Part model, mm, in its own coordinate system. Face numbers are marked on the shaded views. A direction names the side the tool comes from. Coordinates: 2 decimals unless noted, no trailing zeros. Write each loop counter-clockwise with the first axis right and the second up, starting at its lowest first coordinate (ties: lowest second). Pieces come first, ordered by that corner, then holes. Notation, with made-up numbers: (12, -3) -> (71, -3) arc R19 cw to (71, 32) -> close; hole circle Ø7 at (9.5, 22). An arc over 180 degrees is marked (long way). One line per question, with ' | ' between items. Start each with the question number.
Item 1: Saw through at B-B (x = 0). List the corners of the cut face in (y, z).
Item 2: Probe probe 1 along X at (y, z) = (0.85, 0); probe 2 along Z at (x, y) = (0, 1); probe 3 along X at (y, z) = (0.75, -5.5). List the from-to ranges inside material, lowest first. Write a range as [from, to].
Item 3: Two-plate mould, pull along X, no slides. Class the marked faces 1, 2 and 3: pulls with the +X half, pulls with the -X half, needs draft (parallel to the pull), parting line crosses it, or undercut.
Item 4: Saw through at C-C (y = 1.45). List the corners of the cut face in (x, z), and give its area (3 significant figures).
Item 5: 3-axis set-ups, long thin cutter, end or side, ignore diameter. For the marked faces 4 and 5: which of +Z, -Z, +X, -X, +Y, -Y reach the whole face in a straight line?
Item 6: Saw through at A-A (z = 0). List the corners of the cut face in (x, y).
Item 7: Pin check, flat tips, straight feed: pin 1 (2.5 mm diameter, centred on x = 1, z = 8.5, fed in from -Y); pin 2 (0.6 mm diameter, centred on y = 0.5, z = 8, fed in from -X). Stop position of each tip, or through.
from build123d import *

# Parameters (mm, degrees)
SKETCH1_R           = 9.5
BOSS_EXTRUDE1_DEPTH = 2
SKETCH2_R           = 8.05
CUT_EXTRUDE1_DEPTH  = 3
CUT_EXTRUDE2_DEPTH  = 1.2


with BuildPart() as part:
    # Sketch1 → Boss-Extrude1 (new body)
    with BuildSketch(Plane(origin=(0, 0, 0), x_dir=(1, 0, 0), z_dir=(0, 1, 0))):
        Circle(SKETCH1_R)
    extrude(amount=BOSS_EXTRUDE1_DEPTH)

    # Sketch2 → Cut-Extrude1 (cut, through all)
    with BuildSketch(Plane(origin=(0, 2, 0), x_dir=(1, 0, 0), z_dir=(0, 1, 0))):
        Circle(SKETCH2_R)
    extrude(amount=-CUT_EXTRUDE1_DEPTH, mode=Mode.SUBTRACT)

    # Sketch3 → Cut-Extrude2 (cut)
    with BuildSketch(Plane.XZ):
        with BuildLine():
            Line((-3.5, 7.249310312), (-3.5, 8.831760866))
            ThreePointArc((-3.5, 8.831760866), (0, 9.5), (3.5, 8.831760866))
            Line((3.5, 8.831760866), (3.5, 7.249310312))
            ThreePointArc((3.5, 7.249310312), (0, 8.05), (-3.5, 7.249310312))
        make_face()
    extrude(amount=-CUT_EXTRUDE2_DEPTH, mode=Mode.SUBTRACT)


solid = part.part
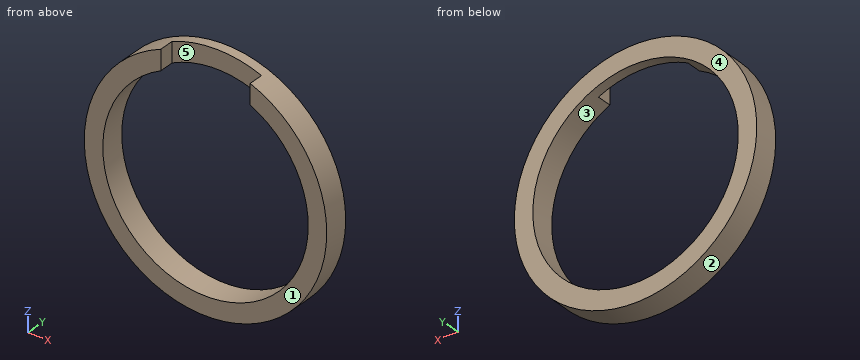
From the geometry:
1) outline: (0, -9.5) -> (2, -9.5) -> (2, -8.05) -> (0, -8.05) -> close; (1.2, 8.05) -> (2, 8.05) -> (2, 9.5) -> (1.2, 9.5) -> close
2) probe 1: [-9.5, -8.05], [8.05, 9.5] | probe 2: [-9.5, -8.05] | probe 3: [-7.75, -5.88], [5.88, 7.75]
3) face 1: needs draft | face 2: parting line crosses it | face 3: undercut
4) outline: circle Ø19 at (0, 0); hole circle Ø16.1 at (0, 0) | area: 79.9 mm2
5) face 4: +Z, -Z, +X, -X, +Y | face 5: +Z, -Y
6) outline: (-9.5, 0) -> (-8.05, 0) -> (-8.05, 2) -> (-9.5, 2) -> close; (8.05, 0) -> (9.5, 0) -> (9.5, 2) -> (8.05, 2) -> close
7) pin 1: y = 1.2 | pin 2: x = -5.56
